```python
from build123d import *

# Parameters (mm, degrees)
RESSALTO_EXTRUS_O1_DEPTH                     = 30
CASCA1_START                                 = -36.5
CASCA1_OUTLINE_W                             = 43
CASCA1_OUTLINE_H                             = 30
CASCA1_DEPTH                                 = 26.5
CASCA1_2_DEPTH                               = 26.5
CASCA1_3_DEPTH                               = 30
CASCA1_4_DEPTH                               = 32
CASCA1_START_2                               = 30
CASCA1_5_DEPTH                               = 2
ESCAREADO_PARA_PARAFUSO_COM_CABE_A_E_2_COUNT = 2
ESCAREADO_PARA_PARAFUSO_COM_CABE_A_E_2_PITCH = 18.308687804


with BuildPart() as part:
    # Esboço1 → Ressalto-extrusão1 (new body)
    with BuildSketch(Plane.XY):
        with BuildLine():
            Line((-10, 0), (-36.5, 0))
            ThreePointArc((-36.5, 0), (-43.571067812, 2.928932188), (-46.5, 10))
            Line((-46.5, 10), (-46.5, 33))
            ThreePointArc((-46.5, 33), (-43.571067812, 40.071067812), (-36.5, 43))
            Line((-36.5, 43), (-10, 43))
            ThreePointArc((-10, 43), (-2.928932188, 40.071067812), (0, 33))
            Line((0, 33), (0, 10))
            ThreePointArc((0, 10), (-2.928932188, 2.928932188), (-10, 0))
        make_face()
    extrude(amount=RESSALTO_EXTRUS_O1_DEPTH)

    # Casca1: read off the stored shape, not the designer's step
    # Casca1 outline → Casca1 (cut)
    with BuildSketch(Plane.YZ.offset(CASCA1_START)):
        with Locations((21.5, 15)):
            Rectangle(CASCA1_OUTLINE_W, CASCA1_OUTLINE_H)
    extrude(amount=CASCA1_DEPTH, mode=Mode.SUBTRACT)

    # Casca1 2 outline → Casca1 2 (add)
    with BuildSketch(Plane.YZ.offset(CASCA1_START)):
        Polygon((-2, 32), (-2, 0), (0, 0), (0, 30), (43, 30), (43, 0), (45, 0), (45, 32), align=None)
    extrude(amount=CASCA1_2_DEPTH)

    # Casca1 3 outline → Casca1 3 (cut)
    with BuildSketch(Plane.XY):
        with BuildLine():
            Line((-36.5, 0), (-36.5, 43))
            ThreePointArc((-36.5, 43), (-43.571067812, 40.071067812), (-46.5, 33))
            Line((-46.5, 33), (-46.5, 10))
            ThreePointArc((-46.5, 10), (-43.571067812, 2.928932188), (-36.5, 0))
        make_face()
        with BuildLine():
            Line((-10, 43), (-10, 0))
            ThreePointArc((-10, 0), (-2.928932188, 2.928932188), (0, 10))
            Line((0, 10), (0, 33))
            ThreePointArc((0, 33), (-2.928932188, 40.071067812), (-10, 43))
        make_face()
    extrude(amount=CASCA1_3_DEPTH, mode=Mode.SUBTRACT)

    # Casca1 4 outline → Casca1 4 (add)
    with BuildSketch(Plane.XY):
        with BuildLine():
            ThreePointArc((-36.5, 45), (-44.985281374, 41.485281374), (-48.5, 33))
            Line((-48.5, 33), (-48.5, 10))
            ThreePointArc((-48.5, 10), (-44.985281374, 1.514718626), (-36.5, -2))
            Line((-36.5, -2), (-36.5, 0))
            ThreePointArc((-36.5, 0), (-43.571067812, 2.928932188), (-46.5, 10))
            Line((-46.5, 10), (-46.5, 33))
            ThreePointArc((-46.5, 33), (-43.571067812, 40.071067812), (-36.5, 43))
            Line((-36.5, 43), (-36.5, 45))
        make_face()
        with BuildLine():
            ThreePointArc((-10, -2), (-1.514718626, 1.514718626), (2, 10))
            Line((2, 10), (2, 33))
            ThreePointArc((2, 33), (-1.514718626, 41.485281374), (-10, 45))
            Line((-10, 45), (-10, 43))
            ThreePointArc((-10, 43), (-2.928932188, 40.071067812), (0, 33))
            Line((0, 33), (0, 10))
            ThreePointArc((0, 10), (-2.928932188, 2.928932188), (-10, 0))
            Line((-10, 0), (-10, -2))
        make_face()
    extrude(amount=CASCA1_4_DEPTH)

    # Casca1 5 outline → Casca1 5 (add)
    with BuildSketch(Plane.XY.offset(CASCA1_START_2)):
        with BuildLine():
            Line((-36.5, 0), (-36.5, 43))
            ThreePointArc((-36.5, 43), (-43.571067812, 40.071067812), (-46.5, 33))
            Line((-46.5, 33), (-46.5, 10))
            ThreePointArc((-46.5, 10), (-43.571067812, 2.928932188), (-36.5, 0))
        make_face()
        with BuildLine():
            Line((-10, 43), (-10, 0))
            ThreePointArc((-10, 0), (-2.928932188, 2.928932188), (0, 10))
            Line((0, 10), (0, 33))
            ThreePointArc((0, 33), (-2.928932188, 40.071067812), (-10, 43))
        make_face()
    extrude(amount=CASCA1_5_DEPTH)

    # Esboço4 → Escareado para parafuso com cabeça escareada chata de M31 (revolve, cut)
    with BuildSketch(Plane(origin=(-32.48511858, 21.158156033, 30), x_dir=(0, 1, 0), z_dir=(1, 0, 0))):
        Polygon((0, 0), (0, 2), (1.7, 2), (1.7, 1.45), (3.15, 0), align=None)
    escareado_para_parafuso_com_cabe_a_escar = revolve(axis=Axis((-32.48511858, 21.158156033, 23.65), (0, 0, 1)), mode=Mode.SUBTRACT)

    # Escareado para parafuso com cabe_a e 2: Escareado para parafuso com cabeça escareada chata de M31 ×2
    with Locations(*[(i * ESCAREADO_PARA_PARAFUSO_COM_CABE_A_E_2_PITCH, 0, 0) for i in range(1, ESCAREADO_PARA_PARAFUSO_COM_CABE_A_E_2_COUNT)]):
        add(escareado_para_parafuso_com_cabe_a_escar, mode=Mode.SUBTRACT)


solid = part.part
```
Model file for the job. Use its own axes, mm. A direction names the side the tool comes from. Coordinates: 2 decimals unless noted, no trailing zeros. Order: outer loops, then holes, each group sorted by start corner. A loop starts at its lowest first (then second) coordinate and runs counter-clockwise, first axis right, second up. Notation, with made-up numbers: (-38, -38.75) - (16, -38.75) arc R19 ccw to (16, -11.75) - close; hole circle Ø6 at (18.5, -30.5). An arc over 180 degrees is marked (long way). Return JSON: item names as keys, results as strings. Group by question number.
1) Flat gauge pins, fed straight in: P1, Ø5.5, axis at x = -14.18, y = 21.16, coming from the +Z side; P2, Ø2, axis at x = -8, z = 16, coming from the +Y side; P3, Ø2, axis at x = -14, y = 37, coming from the -Z side; P4, Ø2.5, axis at x = -32.49, y = 21.16, coming from the -Z side. Where does each tip first touch, or does it go through?
2) Saw through at C-C, the plane y = 12. Write the cut outline in (x, z).
3) Saw through at A-A, the plane z = 11. Write the cut outline in (x, y), plus the area to 3 significant figures.
4) Saw through at B-B, the plane x = -23. Write the cut outline in (y, z), plus the area to 3 significant figures.
5) Mould opens along X. For faces 3 (the cylindrical face through (-33, 22.78, 31.72)), 4 (the cylindrical face through (-44.89, 41.58, 15.78)), 5 (the flat face through (-23, -2, 16)) say: released by +X, released by -X, zero draft, split by the parting line, or undercut.
6) Tool access for faces 1 (the flat face through (-23, 0, 15)), 2 (the cylindrical face through (-1.61, 1.42, 15.78)): list every direction of +Z, -Z, +X, -X, +Y, -Y with a clear straight run to the whole face (end or side of a thin tool).
7) Probe line 1 (Y direction, x = -24, z = 16.5); line 2 (X direction, y = 26.5, z = 10.5); line 3 (Z direction, x = -6.5, y = 14). List the from-to ranges inside material, lowest first. Write a range as from..to.
Values found:
{
 "1": {"P1": "stops at z = 32", "P2": "stops at y = 44.96", "P3": "stops at z = 30", "P4": "passes through"},
 "2": {"outline": "(-48.5, 0) - (-46.5, 0) - (-46.5, 30) - (0, 30) - (0, 0) - (2, 0) - (2, 32) - (-48.5, 32) - close"},
 "3": {"outline": "(-48.5, 10) arc R12 ccw to (-36.5, -2) - (-10, -2) arc R12 ccw to (2, 10) - (2, 33) arc R12 ccw to (-10, 45) - (-36.5, 45) arc R12 ccw to (-48.5, 33) - close; hole (-46.5, 10) arc R10 ccw to (-36.5, 0) - (-10, 0) arc R10 ccw to (0, 10) - (0, 33) arc R10 ccw to (-10, 43) - (-36.5, 43) arc R10 ccw to (-46.5, 33) - close", "area": "336 mm²"},
 "4": {"outline": "(-2, 0) - (0, 0) - (0, 30) - (43, 30) - (43, 0) - (45, 0) - (45, 32) - (-2, 32) - close", "area": "214 mm²"},
 "5": {"face 3": "undercut", "face 4": "released by -X", "face 5": "zero draft"},
 "6": {"face 1": "-Z", "face 2": "+Z, -Z, +X, -Y"},
 "7": {"line 1": "y = -2..0, 43..45", "line 2": "x = -48.5..-46.5, 0..2", "line 3": "z = 30..32"}
}
